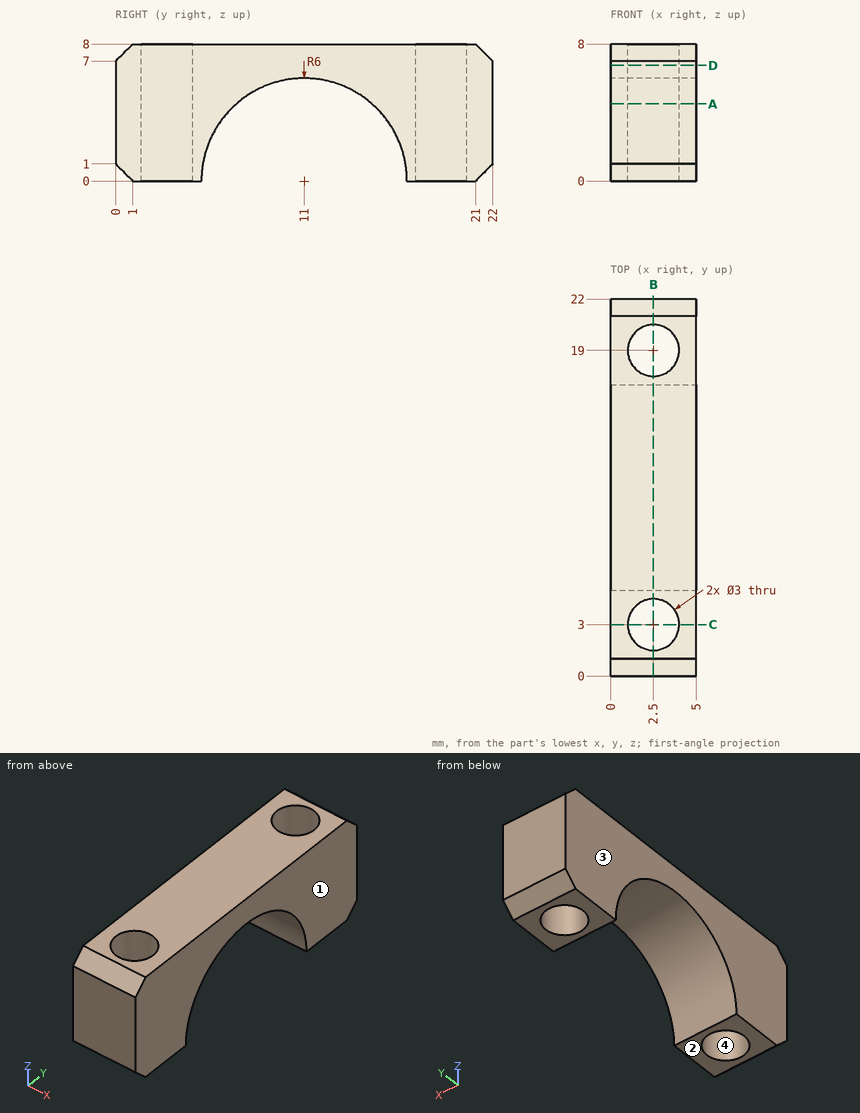
Verification items for this drawing (mm, ordinates from the low corner). Give positions to 0.01 mm unless a question says otherwise; leave off trailing zeros. Loops run counter-clockwise (first coordinate to the right, second up) from the corner with the lowest first, then second, coordinate; pieces in that order, holes last. Notation, with made-up numbers: M 22.25,52 L 28.25,52 A33 ccw 28.25,89 Z; hole C -12,79.5 d10. An arc over 180 degrees is marked long. Write item = value, one per line.
(1) Gauge pin test, flat end, axial feed: pin 1 Ø3 at (x, y) = (3.5, 12) entering from -Z. Record the tip position at first contact, or that the pin passes through.
Answer below:
pin_1 = 5.45
(2) Sectioned sample at C-C, the plane y = 3. Record the cut outline in (x, z).
Answer below:
outline = M 0,0 L 1,0 L 1,8 L 0,8 Z; M 4,0 L 5,0 L 5,8 L 4,8 Z
(3) Material ranges on line 1 (X direction, y = 19, z = 4.5); line 2 (Y direction, x = 3, z = 6.75); line 3 (Y direction, x = 3.5, z = 2.75), recorded low to high. Write a range as [from, to].
Answer below:
line_1 = [0, 1], [4, 5]
line_2 = [0, 1.59], [4.41, 17.59], [20.41, 22]
line_3 = [0, 1.88], [4.12, 5.67], [16.33, 17.88], [20.12, 22]
(4) Release check for a two-part mould opening along X. For the marked faces 1, 2, 3 and 4 record: released by +X, released by -X, zero draft, split by the parting line, or undercut.
Answer below:
face_1 = released by +X
face_2 = zero draft
face_3 = released by -X
face_4 = undercut
(5) Sectioned sample at A-A, the plane z = 4.5. Record the cut outline in (x, y).
Answer below:
outline = M 0,0 L 5,0 L 5,7.03 L 0,7.03 Z; M 0,14.97 L 5,14.97 L 5,22 L 0,22 Z; hole C 2.5,3 d3; hole C 2.5,19 d3
(6) Sectioned sample at B-B, the plane x = 2.5. Record the cut outline in (y, z).
Answer below:
outline = M 0,1 L 1,0 L 1.5,0 L 1.5,8 L 1,8 L 0,7 Z; M 4.5,0 L 5,0 A6 cw 17,0 L 17.5,0 L 17.5,8 L 4.5,8 Z; M 20.5,0 L 21,0 L 22,1 L 22,7 L 21,8 L 20.5,8 Z
(7) Sectioned sample at D-D, the plane z = 6.75. Record the cut outline in (x, y), plus the area to 3 significant figures.
Answer below:
outline = M 0,0 L 5,0 L 5,22 L 0,22 Z; hole C 2.5,3 d3; hole C 2.5,19 d3
area = 95.9 mm2
